For this review, use the dimensioned drawing (mm, ordinates from the lowest corner) and the shaded views. A direction names the side the tool comes from. Give positions to 0.01 mm unless a question says otherwise; leave off trailing zeros. Write each loop counter-clockwise with the first axis right and the second up, starting at its lowest first coordinate (ties: lowest second). Pieces come first, ordered by that corner, then holes.
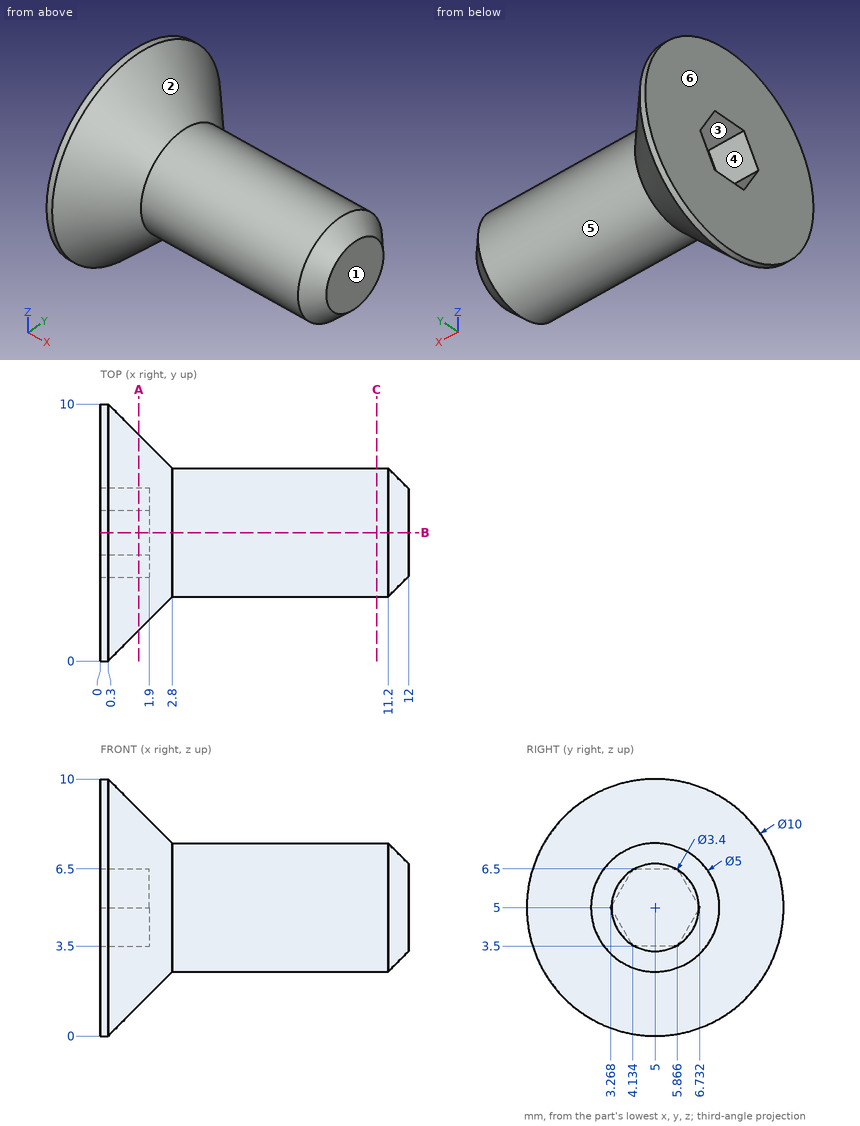
(1) We need section A-A (x = 1.5). Write out the cut boundary in (y, z).
(2) Tool access review of the marked faces 4, 5 and 6: name each direction out of +Z, -Z, +X, -X, +Y, -Y from which nothing blocks a thin tool from reaching the whole face with its end or side.
(3) Clearance check with flat-ended pins moving along their axes: pin 1 Ø0.9 at (x, y) = (1.5, 5) entering from -Z; pin 2 Ø6 at (x, y) = (6.5, 2) entering from -Z; pin 3 Ø5 at (x, z) = (7, 2) entering from +Y; pin 4 Ø5 at (y, z) = (5.5, 8.5) entering from -X. State where each tip first meets the part, or that it passes through.
(4) We need section B-B (y = 5). Write out the cut boundary in (x, z).
(5) We need section C-C (x = 10.75). Write out the cut boundary in (y, z).
(6) The part is to be moulded in two halves that separate along Y. For the marked faces 1, 2 and 3, say which applies: +Y half, -Y half, draft (parallel to the pull), parting line (faces both ways), or undercut.
(7) For L1, parallel to Z at x = 3.75, y = 7; L2, parallel to Z at x = 8.5, y = 5, list the stretches that pass through material, from the lowest coordinate up.
The answers:
1. outline: circle Ø7.6 at (5, 5); hole (3.27, 5) - (4.13, 3.5) - (5.87, 3.5) - (6.73, 5) - (5.87, 6.5) - (4.13, 6.5) - close
2. face 4: -X
2. face 5: +X
2. face 6: +Z, -Z, -X, +Y, -Y
3. pin 1: stops at z = 0.75
3. pin 2: stops at z = 2.5
3. pin 3: stops at y = 7.45
3. pin 4: stops at x = 0
4. outline: (0, 0) - (0.3, 0) - (2.8, 2.5) - (11.2, 2.5) - (12, 3.3) - (12, 6.7) - (11.2, 7.5) - (2.8, 7.5) - (0.3, 10) - (0, 10) - (0, 6.5) - (1.9, 6.5) - (1.9, 3.5) - (0, 3.5) - close
5. outline: circle Ø5 at (5, 5)
6. face 1: draft
6. face 2: parting line
6. face 3: undercut
7. L1: z = 3.5 to 6.5
7. L2: z = 2.5 to 7.5
